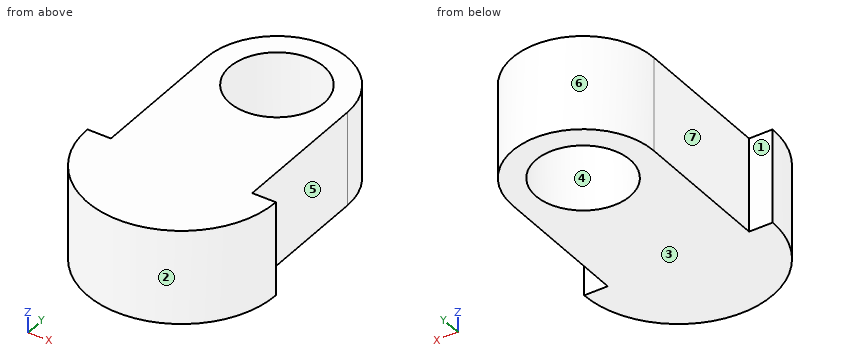
Autodesk Inventor part; units mm, degrees
ref_plane "YZ Plane" through (0, 0, 0) normal (1, 0, 0) x (0, 1, 0)
ref_plane "XZ Plane" through (0, 0, 0) normal (0, 1, 0) x (-1, 0, 0)
ref_plane "XY Plane" through (0, 0, 0) normal (0, 0, 1) x (1, 0, 0)
sketch "Sketch1" plane through (0, 0, 0) normal (0, 0, 1) x (1, 0, 0)
  line L0 (-6, 0) -> (-6, 12)
  line L1 (-8, 0) -> (-6, 0)
  line L2 (8, 0) -> (6, 0)
  line L3 (6, 0) -> (6, 12)
  arc A0 (-8, 0) -> (8, 0) centre (0, 0) ccw
  arc A1 (6, 12) -> (-6, 12) centre (0, 12) ccw
  circle A2 centre (0, 12) radius 4
  point P0 (0, -8)
  dimension "d1" = 2
  dimension "d2" = 8
  dimension "d3" = 2
  dimension "d9" = 20
extrude "Extrusion1" add sketch "Sketch1" along normal blind 8
properties part number "khurramf_01_Swing"
Can you work these out from the model? Positions are in its coordinate system, mm. Face numbers are marked on the shaded views. A direction names the side the tool comes from. Round coordinates to 2 decimals unless told otherwise and drop trailing zeros. Order: outer loops, then holes, each group sorted by start corner. A loop starts at its lowest first (then second) coordinate and runs counter-clockwise, first axis right, second up. Notation, with made-up numbers: (67.5, 58.25) -> (82.5, 58.25) arc R10 ccw to (82.5, 69.25) -> close; hole circle Ø11 at (-0.75, 69). An arc over 180 degrees is marked (long way). Return JSON: item names as keys, results as strings. Group by question number.
1. If we section it at C-C, the plane z = 4.5: Write out the boundary of the cut face in (x, y).
2. I need wall thicknesses on line 1 (Y direction, x = 0, z = 2); line 2 (X direction, y = 5.75, z = 3.25); line 3 (X direction, y = 14, z = 5.5). Which ranges of each line are inside material? Lowest first, please. Write a range as [from, to].
3. If we section it at B-B, the plane y = 9.25: Write out the boundary of the cut face in (x, z).
4. If we section it at D-D, the plane y = 4.25: Write out the boundary of the cut face in (x, z).
5. Will these pins go through, and if not, where does the flat tip stop? pin 1 (0.6 mm diameter, centred on x = 6.5, z = 5, fed in from +Y); pin 2 (3 mm diameter, centred on x = -4, y = 13, fed in from -Z); pin 3 (2 mm diameter, centred on x = -5, z = 4.5, fed in from +Y); pin 4 (5 mm diameter, centred on x = 0, y = 12, fed in from +Z) (3 decimals).
6. We'd pull the mould along Y, two halves only. Please class the marked faces 1, 2, 3 and 4: released by +Y, released by -Y, zero draft, split by the parting line, or undercut.
7. If we section it at A-A, the plane x = 0: Write out the boundary of the cut face in (y, z).
8. Which directions (+Z, -Z, +X, -X, +Y, -Y) give clear straight access to the entire face, cutting with the end or side of a thin tool? Please do the marked faces 5, 6 and 7.
Output values:
{
 "1": {"outline": "(-8, 0) arc R8 ccw to (8, 0) -> (6, 0) -> (6, 12) arc R6 ccw to (-6, 12) -> (-6, 0) -> close; hole circle Ø8 at (0, 12)"},
 "2": {"line 1": "[-8, 8], [16, 18]", "line 2": "[-6, 6]", "line 3": "[-5.66, -3.46], [3.46, 5.66]"},
 "3": {"outline": "(-6, 0) -> (-2.9, 0) -> (-2.9, 8) -> (-6, 8) -> close; (2.9, 0) -> (6, 0) -> (6, 8) -> (2.9, 8) -> close"},
 "4": {"outline": "(-6, 0) -> (6, 0) -> (6, 8) -> (-6, 8) -> close"},
 "5": {"pin 1": "y = 0", "pin 2": "z = 0", "pin 3": "y = 16.47", "pin 4": "through"},
 "6": {"face 1": "released by +Y", "face 2": "released by -Y", "face 3": "zero draft", "face 4": "undercut"},
 "7": {"outline": "(-8, 0) -> (8, 0) -> (8, 8) -> (-8, 8) -> close; (16, 0) -> (18, 0) -> (18, 8) -> (16, 8) -> close"},
 "8": {"face 5": "+Z, -Z, +X, +Y", "face 6": "+Z, -Z, +Y", "face 7": "+Z, -Z, -X, +Y"}
}
